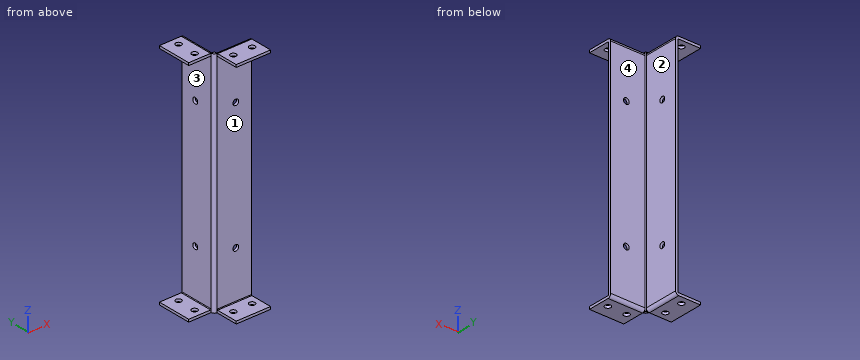
```python
from build123d import *

# Parameters (mm, degrees)
SKETCH1_W                      = 60
SKETCH1_H                      = 364.5
BASE_FLANGE1_DEPTH             = 4
EDGE_FLANGE1_STRIP_W           = 18
EDGE_FLANGE1_STRIP_H           = 4
EDGE_FLANGE1_STRIP_CUT_DEPTH   = 364.5
EDGE_FLANGE1_DEPTH             = 364.5
EDGE_FLANGE2_STRIP_W           = 18
EDGE_FLANGE2_STRIP_H           = 4
EDGE_FLANGE2_STRIP_CUT_DEPTH   = 55
EDGE_FLANGE2_STRIP_2_W         = 18
EDGE_FLANGE2_STRIP_2_H         = 4
EDGE_FLANGE2_STRIP_CUT_2_DEPTH = 55
EDGE_FLANGE2_STRIP_3_W         = 18
EDGE_FLANGE2_STRIP_3_H         = 4
EDGE_FLANGE2_STRIP_CUT_3_DEPTH = 55
EDGE_FLANGE2_STRIP_4_W         = 18
EDGE_FLANGE2_STRIP_4_H         = 4
EDGE_FLANGE2_STRIP_CUT_4_DEPTH = 55
EDGE_FLANGE2_DEPTH             = 55
EDGE_FLANGE2_BEND_DEPTH        = 55
EDGE_FLANGE2_BEND_2_DEPTH      = 55
EDGE_FLANGE2_BEND_3_DEPTH      = 55
SKETCH18_R                     = 4.6
EXTRUDE1_DEPTH                 = 376.254913359
SKETCH19_R                     = 4.6
EXTRUDE2_DEPTH                 = 4
SKETCH20_R                     = 4.6
EXTRUDE3_DEPTH                 = 4


# Sheet-metal steps are written as plain solids
with BuildPart() as part:
    # Sketch1 → Base-Flange1 (new body)
    with BuildSketch(Plane(origin=(0, 0, 0), x_dir=(1, 0, 0), z_dir=(0, 1, 0))):
        Rectangle(SKETCH1_W, SKETCH1_H)
    extrude(amount=BASE_FLANGE1_DEPTH)

    # Edge-Flange1 strip (across the edge) → Edge-Flange1 strip cut (cut)
    with BuildSketch(Plane(origin=(-30, 4, -182.25), x_dir=(1, 0, 0), z_dir=(0, 0, 1))):
        with Locations((-4, -2)):
            Rectangle(EDGE_FLANGE1_STRIP_W, EDGE_FLANGE1_STRIP_H)
    extrude(amount=EDGE_FLANGE1_STRIP_CUT_DEPTH, mode=Mode.SUBTRACT)

    # Edge-Flange1 section (across the edge) → Edge-Flange1 (add)
    with BuildSketch(Plane(origin=(-30, 4, -182.25), x_dir=(1, 0, 0), z_dir=(0, 0, 1))):
        with BuildLine():
            Line((0, 1), (0, 56))
            Line((0, 56), (4, 56))
            Line((4, 56), (4, 1))
            ThreePointArc((4, 1), (4.292893219, 0.292893219), (5, 0))
            Line((5, 0), (5, -4))
            ThreePointArc((5, -4), (1.464466094, -2.535533906), (0, 1))
        make_face()
    extrude(amount=EDGE_FLANGE1_DEPTH)

    # Edge-Flange2 strip (across the edge) → Edge-Flange2 strip cut (cut)
    with BuildSketch(Plane(origin=(-30, 5, 182.25), x_dir=(0, 0, -1), z_dir=(0, 1, 0))):
        with Locations((-4, -2)):
            Rectangle(EDGE_FLANGE2_STRIP_W, EDGE_FLANGE2_STRIP_H)
    extrude(amount=EDGE_FLANGE2_STRIP_CUT_DEPTH, mode=Mode.SUBTRACT)

    # Edge-Flange2 strip 2 (across the edge) → Edge-Flange2 strip cut 2 (cut)
    with BuildSketch(Plane(origin=(30, 0, 182.25), x_dir=(0, 0, -1), z_dir=(-1, 0, 0))):
        with Locations((-4, -2)):
            Rectangle(EDGE_FLANGE2_STRIP_2_W, EDGE_FLANGE2_STRIP_2_H)
    extrude(amount=EDGE_FLANGE2_STRIP_CUT_2_DEPTH, mode=Mode.SUBTRACT)

    # Edge-Flange2 strip 3 (across the edge) → Edge-Flange2 strip cut 3 (cut)
    with BuildSketch(Plane(origin=(-30, 60, -182.25), x_dir=(0, 0, 1), z_dir=(0, -1, 0))):
        with Locations((-4, -2)):
            Rectangle(EDGE_FLANGE2_STRIP_3_W, EDGE_FLANGE2_STRIP_3_H)
    extrude(amount=EDGE_FLANGE2_STRIP_CUT_3_DEPTH, mode=Mode.SUBTRACT)

    # Edge-Flange2 strip 4 (across the edge) → Edge-Flange2 strip cut 4 (cut)
    with BuildSketch(Plane(origin=(-25, 0, -182.25), x_dir=(0, 0, 1), z_dir=(1, 0, 0))):
        with Locations((-4, -2)):
            Rectangle(EDGE_FLANGE2_STRIP_4_W, EDGE_FLANGE2_STRIP_4_H)
    extrude(amount=EDGE_FLANGE2_STRIP_CUT_4_DEPTH, mode=Mode.SUBTRACT)

    # Edge-Flange2 section (across the edge) → Edge-Flange2 (add)
    with BuildSketch(Plane(origin=(-30, 5, 182.25), x_dir=(0, 0, -1), z_dir=(0, 1, 0))):
        with BuildLine():
            Line((0, 1), (0, 36))
            Line((0, 36), (4, 36))
            Line((4, 36), (4, 1))
            ThreePointArc((4, 1), (4.292893219, 0.292893219), (5, 0))
            Line((5, 0), (5, -4))
            ThreePointArc((5, -4), (1.464466094, -2.535533906), (0, 1))
        make_face()
    extrude(amount=EDGE_FLANGE2_DEPTH)

    # Edge-Flange2 section 2 (across the edge) → Edge-Flange2 bend (add)
    with BuildSketch(Plane(origin=(30, 0, 182.25), x_dir=(0, 0, -1), z_dir=(-1, 0, 0))):
        with BuildLine():
            Line((0, 1), (0, 36))
            Line((0, 36), (4, 36))
            Line((4, 36), (4, 1))
            ThreePointArc((4, 1), (4.292893219, 0.292893219), (5, 0))
            Line((5, 0), (5, -4))
            ThreePointArc((5, -4), (1.464466094, -2.535533906), (0, 1))
        make_face()
    extrude(amount=EDGE_FLANGE2_BEND_DEPTH)

    # Edge-Flange2 section 3 (across the edge) → Edge-Flange2 bend 2 (add)
    with BuildSketch(Plane(origin=(-30, 60, -182.25), x_dir=(0, 0, 1), z_dir=(0, -1, 0))):
        with BuildLine():
            Line((0, 1), (0, 36))
            Line((0, 36), (4, 36))
            Line((4, 36), (4, 1))
            ThreePointArc((4, 1), (4.292893219, 0.292893219), (5, 0))
            Line((5, 0), (5, -4))
            ThreePointArc((5, -4), (1.464466094, -2.535533906), (0, 1))
        make_face()
    extrude(amount=EDGE_FLANGE2_BEND_2_DEPTH)

    # Edge-Flange2 section 4 (across the edge) → Edge-Flange2 bend 3 (add)
    with BuildSketch(Plane(origin=(-25, 0, -182.25), x_dir=(0, 0, 1), z_dir=(1, 0, 0))):
        with BuildLine():
            Line((0, 1), (0, 36))
            Line((0, 36), (4, 36))
            Line((4, 36), (4, 1))
            ThreePointArc((4, 1), (4.292893219, 0.292893219), (5, 0))
            Line((5, 0), (5, -4))
            ThreePointArc((5, -4), (1.464466094, -2.535533906), (0, 1))
        make_face()
    extrude(amount=EDGE_FLANGE2_BEND_3_DEPTH)

    # Sketch18 → Extrude1 (cut, through all)
    with BuildSketch(Plane.XY.offset(182.25)):
        with Locations((-46, 47.5)):
            Circle(SKETCH18_R)
        with Locations((-46, 17.5)):
            Circle(SKETCH18_R)
        with Locations((-12.5, -16)):
            Circle(SKETCH18_R)
        with Locations((17.5, -16)):
            Circle(SKETCH18_R)
    extrude(amount=-EXTRUDE1_DEPTH, mode=Mode.SUBTRACT)

    # Sketch19 → Extrude2 (cut)
    with BuildSketch(Plane(origin=(-26, 0, 0), x_dir=(0, 0, -1), z_dir=(1, 0, 0))):
        with Locations(Location((-102.25, 35, 0), (0, 0, 90))):
            Circle(SKETCH19_R)
        with Locations(Location((102.25, 35, 0), (0, 0, 90))):
            Circle(SKETCH19_R)
    extrude(amount=-EXTRUDE2_DEPTH, mode=Mode.SUBTRACT)

    # Sketch20 → Extrude3 (cut)
    with BuildSketch(Plane(origin=(0, 4, 0), x_dir=(1, 0, 0), z_dir=(0, 1, 0))):
        with Locations(Location((5, 102.25, 0), (0, 0, 270))):
            Circle(SKETCH20_R)
        with Locations(Location((5, -102.25, 0), (0, 0, 270))):
            Circle(SKETCH20_R)
    extrude(amount=-EXTRUDE3_DEPTH, mode=Mode.SUBTRACT)


solid = part.part
```
Work out the finished part from the listing and answer in its coordinate system (mm). Face numbers are marked on the shaded views. A direction names the side the tool comes from. Give positions to 0.01 mm unless a question says otherwise; leave off trailing zeros. Order: outer loops, then holes, each group sorted by start corner. A loop starts at its lowest first (then second) coordinate and runs counter-clockwise, first axis right, second up. Notation, with made-up numbers: M 28,-5 L 53,-5 A23 cw 53,4 Z; hole C 28.25,0 d9. An arc over 180 degrees is marked long. Return JSON: item names as keys, results as strings.
1) For a pull along Z with two mould halves and no side action, classify the marked faces 3 and 4 as +Z half, -Z half, draft (parallel to the pull), parting line (faces both ways), or undercut.
Resolved:
{"face 3": "undercut", "face 4": "draft"}
2) Each of these flat-tipped pins is pushed along its axis until it touches: pin 1 (12 mm diameter, centred on y = 35, z = -102.25, fed in from -X); pin 2 (5.5 mm diameter, centred on y = -26.5, z = -180, fed in from -X); pin 3 (8.5 mm diameter, centred on x = 17.5, y = -16, fed in from -Z); pin 4 (6 mm diameter, centred on x = -18.5, z = 6, fed in from -Y). Where does it stop, or does it pass through?
Resolved:
{"pin 1": "x = -30", "pin 2": "x = -25", "pin 3": "through", "pin 4": "y = 0"}
3) Section C-C, the plane x = 17.5 is taken. Write down the section's boundary in (y, z), plus the area to 3 significant figures.
Resolved:
{"outline": "M -36,-182.25 L -20.6,-182.25 L -20.6,-178.25 L -36,-178.25 Z; M -36,178.25 L -20.6,178.25 L -20.6,182.25 L -36,182.25 Z; M -11.4,-182.25 L -1,-182.25 A5 ccw 4,-177.25 L 4,177.25 A5 ccw -1,182.25 L -11.4,182.25 L -11.4,178.25 L -1,178.25 A1 cw 0,177.25 L 0,-177.25 A1 cw -1,-178.25 L -11.4,-178.25 Z", "area": "1,660 mm^2"}
4) Section B-B, the plane x = -38 is taken. Write down the section's boundary in (y, z).
Resolved:
{"outline": "M 5,-182.25 L 60,-182.25 L 60,-178.25 L 5,-178.25 Z; M 5,178.25 L 60,178.25 L 60,182.25 L 5,182.25 Z"}
5) Section D-D, the plane y = -16 is taken. Write down the section's boundary in (x, z).
Resolved:
{"outline": "M -25,-182.25 L -17.1,-182.25 L -17.1,-178.25 L -25,-178.25 Z; M -25,178.25 L -17.1,178.25 L -17.1,182.25 L -25,182.25 Z; M -7.9,-182.25 L 12.9,-182.25 L 12.9,-178.25 L -7.9,-178.25 Z; M -7.9,178.25 L 12.9,178.25 L 12.9,182.25 L -7.9,182.25 Z; M 22.1,-182.25 L 30,-182.25 L 30,-178.25 L 22.1,-178.25 Z; M 22.1,178.25 L 30,178.25 L 30,182.25 L 22.1,182.25 Z"}
6) Straight lines are drawn through the part: line 1 along Y through (x, z) = (-46, -179.85); line 2 along X through (y, z) = (52.5, 94); line 3 along Z through (x, y) = (-53, 13.5). For each, find the intervals that lie inside material, in ascending order. Write a range as [from, to].
Resolved:
{"line 1": "[5, 12.9], [22.1, 42.9], [52.1, 60]", "line 2": "[-30, -26]", "line 3": "[-182.25, -178.25], [178.25, 182.25]"}
7) Section A-A, the plane y = 35 is taken. Write down the section's boundary in (x, z).
Resolved:
{"outline": "M -66,-182.25 L -31,-182.25 A5 ccw -26,-177.25 L -26,-106.85 L -30,-106.85 L -30,-177.25 A1 cw -31,-178.25 L -66,-178.25 Z; M -66,178.25 L -31,178.25 A1 cw -30,177.25 L -30,106.85 L -26,106.85 L -26,177.25 A5 ccw -31,182.25 L -66,182.25 Z; M -30,-97.65 L -26,-97.65 L -26,97.65 L -30,97.65 Z"}
8) A tool of negligible diameter and unlimited length cuts with its end or side. For the marked faces 1 and 2, from which of +Z, -Z, +X, -X, +Y, -Y can it reach the whole face along a straight path? Write none if from no direction.
Resolved:
{"face 1": "+X, -X, -Y", "face 2": "+Z, -Z, +X, +Y"}
